Check sheet for the drawn part. Datum: minimum x, y, z corner. Units: mm. Round coordinates to 2 decimals unless told otherwise and drop trailing zeros. Loops run counter-clockwise (first coordinate to the right, second up) from the corner with the lowest first, then second, coordinate; pieces in that order, holes last. Notation, with made-up numbers: (14, 16) -> (28, 16) arc R32 cw to (28, 50) -> close; hole circle Ø11 at (66, 63). An arc over 180 degrees is marked (long way). Use CSV: the item, a comma, the result in double quotes. Start each with the question number.
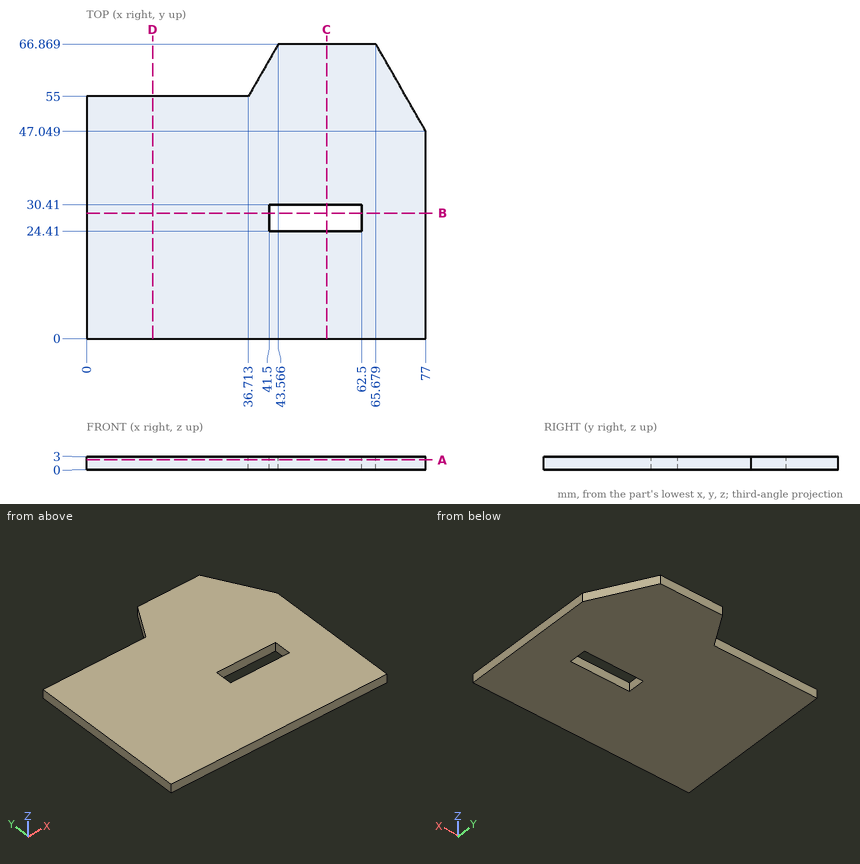
Q1. Thickness scan on L1, parallel to Y at x = 49.5, z = 2.1; L2, parallel to X at y = 29, z = 0.9; L3, parallel to Y at x = 7.5, z = 1.55. Record the ranges inside material, lowest first. Write a range as from..to.
Q2. Cross-section at B-B (y = 28.5). Record the boundary of the cut face in (x, z).
Q3. Cross-section at D-D (x = 15). Record the boundary of the cut face in (y, z), and give its area (3 significant figures).
Q4. Cross-section at C-C (x = 54.5). Record the boundary of the cut face in (y, z).
Q5. Cross-section at A-A (z = 2.3). Record the boundary of the cut face in (x, y), and give its area (3 significant figures).
Answer list:
1,L1,"y = 0..24.41, 30.41..66.87"
1,L2,"x = 0..41.5, 62.5..77"
1,L3,"y = 0..55"
2,outline,"(0, 0) -> (41.5, 0) -> (41.5, 3) -> (0, 3) -> close; (62.5, 0) -> (77, 0) -> (77, 3) -> (62.5, 3) -> close"
3,outline,"(0, 0) -> (55, 0) -> (55, 3) -> (0, 3) -> close"
3,area,"165 mm2"
4,outline,"(0, 0) -> (24.41, 0) -> (24.41, 3) -> (0, 3) -> close; (30.41, 0) -> (66.87, 0) -> (66.87, 3) -> (30.41, 3) -> close"
5,outline,"(0, 0) -> (77, 0) -> (77, 47.05) -> (65.68, 66.87) -> (43.57, 66.87) -> (36.71, 55) -> (0, 55) -> close; hole (41.5, 24.41) -> (62.5, 24.41) -> (62.5, 30.41) -> (41.5, 30.41) -> close"
5,area,"4,430 mm2"
